Build history of the part. All positions in model axes, mm. Give positions to 0.01 mm unless a question says otherwise; leave off trailing zeros. Loops run counter-clockwise (first coordinate to the right, second up) from the corner with the lowest first, then second, coordinate; pieces in that order, holes last. Notation, with made-up numbers: M 50,8.25 L 109,8.25 A34 ccw 109,43.25 Z; hole C -8.75,-28.5 d4. An arc over 180 degrees is marked long. Put each result on its own line as item: value.
```python
from build123d import *

# Parameters (mm, degrees)
SKETCH5_W             = 500
SKETCH5_H             = 300
BOSS_EXTRUDE1_DEPTH   = 12
SKETCH5_H_2           = 224
BOSS_EXTRUDE1_2_DEPTH = 12
BOSS_EXTRUDE1_3_DEPTH = 12
SKETCH5_3_W           = 500
SKETCH5_3_H           = 14
BOSS_EXTRUDE2_DEPTH   = 6
SKETCH5_4_W           = 500
SKETCH5_4_H           = 12
BOSS_EXTRUDE3_DEPTH   = 12
CHAMFER1_SIZE         = 12


with BuildPart() as part:
    # Sketch5 → Boss-Extrude1 (new body)
    with BuildSketch(Plane(origin=(0, 0, 0), x_dir=(1, 0, 0), z_dir=(0, 1, 0))):
        with Locations((250, 400)):
            Rectangle(SKETCH5_W, SKETCH5_H)
    extrude(amount=BOSS_EXTRUDE1_DEPTH)



with BuildPart() as body_2:
    # Sketch5 → Boss-Extrude1 2 (new body)
    with BuildSketch(Plane(origin=(0, 0, 0), x_dir=(1, 0, 0), z_dir=(0, 1, 0))):
        with Locations((250, 124)):
            Rectangle(SKETCH5_W, SKETCH5_H_2)
    extrude(amount=BOSS_EXTRUDE1_2_DEPTH)


with BuildPart() as body_3:
    # Sketch5 → Boss-Extrude1 3 (new body)
    with BuildSketch(Plane(origin=(0, 0, 0), x_dir=(1, 0, 0), z_dir=(0, 1, 0))):
        with Locations((250, 676)):
            Rectangle(SKETCH5_W, SKETCH5_H_2)
    extrude(amount=BOSS_EXTRUDE1_3_DEPTH)


with BuildPart() as part_1:
    add(part.part)

    add(body_2.part)  # Boss-Extrude2 merges body 2

    add(body_3.part)  # Boss-Extrude2 merges body 3
    # Sketch5<3> → Boss-Extrude2 (add)
    with BuildSketch(Plane(origin=(0, 0, 0), x_dir=(1, 0, 0), z_dir=(0, 1, 0))):
        with Locations((250, 243)):
            Rectangle(SKETCH5_3_W, SKETCH5_3_H)
        with Locations((250, 557)):
            Rectangle(SKETCH5_3_W, SKETCH5_3_H)
    extrude(amount=BOSS_EXTRUDE2_DEPTH)

    # Sketch5<4> → Boss-Extrude3 (add)
    with BuildSketch(Plane(origin=(0, 0, 0), x_dir=(1, 0, 0), z_dir=(0, 1, 0))):
        with Locations((250, 6)):
            Rectangle(SKETCH5_4_W, SKETCH5_4_H)
        with Locations((250, 794)):
            Rectangle(SKETCH5_4_W, SKETCH5_4_H)
    extrude(amount=BOSS_EXTRUDE3_DEPTH)

    # Chamfer1
    # the kernel refuses this chamfer: 12 mm, written as the material it takes off along each edge
    with BuildSketch(Plane(origin=(0, 12, -580.860195856), x_dir=(-0.027495876610586372, -0.9996219169112968, 0), z_dir=(0, 0, 1)), Plane(origin=(500, 12, -219.139804144), x_dir=(0.027495876610586778, -0.9996219169112968, 0), z_dir=(0, 0, -1))) as chamfer1_piece_1:
        Polygon((CHAMFER1_SIZE * 0.999621916911, CHAMFER1_SIZE * 0.0274958766106), (-CHAMFER1_SIZE * 0.0274958766106, CHAMFER1_SIZE * 0.999621916911), (0, 0), align=None)
    extrude(amount=361.720391711, mode=Mode.SUBTRACT)
    with BuildSketch(Plane(origin=(0, 12, 30.860195856), x_dir=(-0.027495876610586372, -0.9996219169112968, 0), z_dir=(0, 0, -1)), Plane(origin=(0, 12, -533.139804144), x_dir=(-0.027495876610586372, -0.9996219169112968, 0), z_dir=(0, 0, -1))) as chamfer1_piece_2:
        Polygon((CHAMFER1_SIZE * 0.999621916911, -CHAMFER1_SIZE * 0.0274958766106), (-CHAMFER1_SIZE * 0.0274958766106, -CHAMFER1_SIZE * 0.999621916911), (0, 0), align=None)
    extrude(amount=297.720391711, mode=Mode.SUBTRACT)
    with BuildSketch(Plane(origin=(500, 12, 30.860195856), x_dir=(0.027495876610586778, -0.9996219169112968, 0), z_dir=(0, 0, -1)), Plane(origin=(500, 12, -533.139804144), x_dir=(0.027495876610586778, -0.9996219169112968, 0), z_dir=(0, 0, -1))) as chamfer1_piece_3:
        Polygon((CHAMFER1_SIZE * 0.999621916911, CHAMFER1_SIZE * 0.0274958766106), (-CHAMFER1_SIZE * 0.0274958766106, CHAMFER1_SIZE * 0.999621916911), (0, 0), align=None)
    extrude(amount=297.720391711, mode=Mode.SUBTRACT)
    with BuildSketch(Plane(origin=(-30.860195856, 12, 0), x_dir=(0, -0.9996219169112968, 0.027495876610586372), z_dir=(1, 0, 0))) as chamfer1_piece_4:
        Polygon((CHAMFER1_SIZE * 0.999621916911, CHAMFER1_SIZE * 0.0274958766106), (-CHAMFER1_SIZE * 0.0274958766106, CHAMFER1_SIZE * 0.999621916911), (0, 0), align=None)
    extrude(amount=561.720391711, mode=Mode.SUBTRACT)
    with BuildSketch(Plane(origin=(530.860195856, 12, -800), x_dir=(0, 0.027495876610586462, 0.9996219169112968), z_dir=(-1, 0, 0))) as chamfer1_piece_5:
        Polygon((CHAMFER1_SIZE * 0.999621916911, -CHAMFER1_SIZE * 0.0274958766106), (-CHAMFER1_SIZE * 0.0274958766106, -CHAMFER1_SIZE * 0.999621916911), (0, 0), align=None)
    extrude(amount=561.720391711, mode=Mode.SUBTRACT)


solid = part_1.part
```
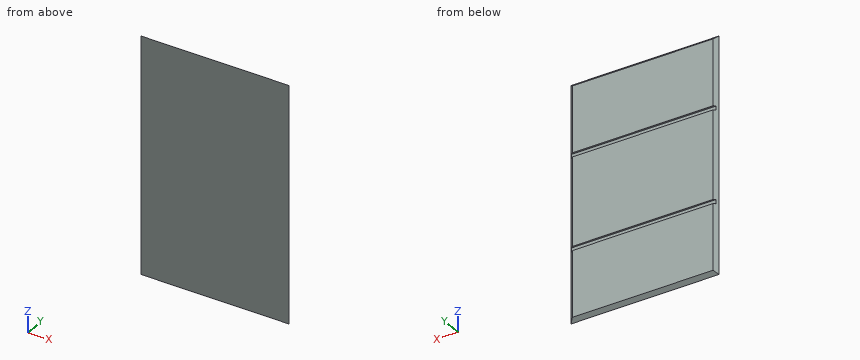
Q1. Slice it at A-A (x = 420). List the corners of the cut face in (y, z), and give its area (3 significant figures).
Here are the results:
outline: M 0,-800 L 12,-788 L 12,-564 L 6,-564 L 6,-550 L 12,-550 L 12,-250 L 6,-250 L 6,-236 L 12,-236 L 12,-12 L 0,0 Z
area: 9,290 mm²
Q2. Slice it at C-C (z = -653). List the corners of the cut face in (x, y), and give its area (3 significant figures).
Here are the results:
outline: M 0,0 L 500,0 L 488,12 L 12,12 Z
area: 5,860 mm²
Q3. Probe line 1 (Z direction, x = 452.5, y = 8.5); line 2 (Z direction, x = 292, y = 6.25); line 3 (Z direction, x = 439, y = 2.25). List the from-to ranges inside material, lowest first. Write a range as from..to.
Here are the results:
line 1: -791.5..-564, -550..-250, -236..-8.5
line 2: -793.75..-564, -550..-250, -236..-6.25
line 3: -797.75..-2.25
Q4. Slice it at B-B (y = 3.5). List the corners of the cut face in (x, z), and give its area (3 significant figures).
Here are the results:
outline: M 3.5,-796.5 L 496.5,-796.5 L 496.5,-3.5 L 3.5,-3.5 Z
area: 391,000 mm²
Q5. Drop flat-ended pins along their axis: pin 1 Ø7 at (x, z) = (304, -554.5) entering from +Y; pin 2 Ø3 at (x, y) = (341, 8.5) entering from +Z; pin 3 Ø6 at (x, y) = (262, 9.5) entering from +Z. Give the stop position or say it passes through.
Here are the results:
pin 1: y = 6
pin 2: z = -7
pin 3: z = -6.5
